Here's the drawing with two shaded views (mm, measured from the low corner). I have some questions. Round coordinates to 2 decimals unless told otherwise and drop trailing zeros. Loops run counter-clockwise (first coordinate to the right, second up) from the corner with the lowest first, then second, coordinate; pieces in that order, holes last. Notation, with made-up numbers: (-5, 45.25) -> (51, 45.25) arc R23 ccw to (51, 76.25) -> close; hole circle Ø3 at (75.5, -29). An arc over 180 degrees is marked (long way). Write each question's results on one line, items separated by ' | '. Start each with the question number.
1) Imagine slicing it at C-C, the plane z = 2.15. List the corners of the cut face in (x, y) for me, plus the area to 3 significant figures.
2) Imagine slicing it at B-B, the plane x = 95. List the corners of the cut face in (y, z) for me, plus the area to 3 significant figures.
3) For P1, Ø3.5, axis at x = 5, y = 5, coming from the +Z side, with a flat end and sliding along its axis, tell me the tip position at first contact or that it passes through.
4) Imagine slicing it at A-A, the plane y = 5. List the corners of the cut face in (x, z) for me, plus the area to 3 significant figures.
5) Imagine slicing it at D-D, the plane x = 75. List the corners of the cut face in (y, z) for me, plus the area to 3 significant figures.
6) If I drill on probe 1 along Y at (x, z) = (95, 1.8); probe 2 along X at (y, z) = (50, 0.8); probe 3 along X at (y, z) = (27.5, 2.25), over which ranges is the centre line in solid material (lowest first)?
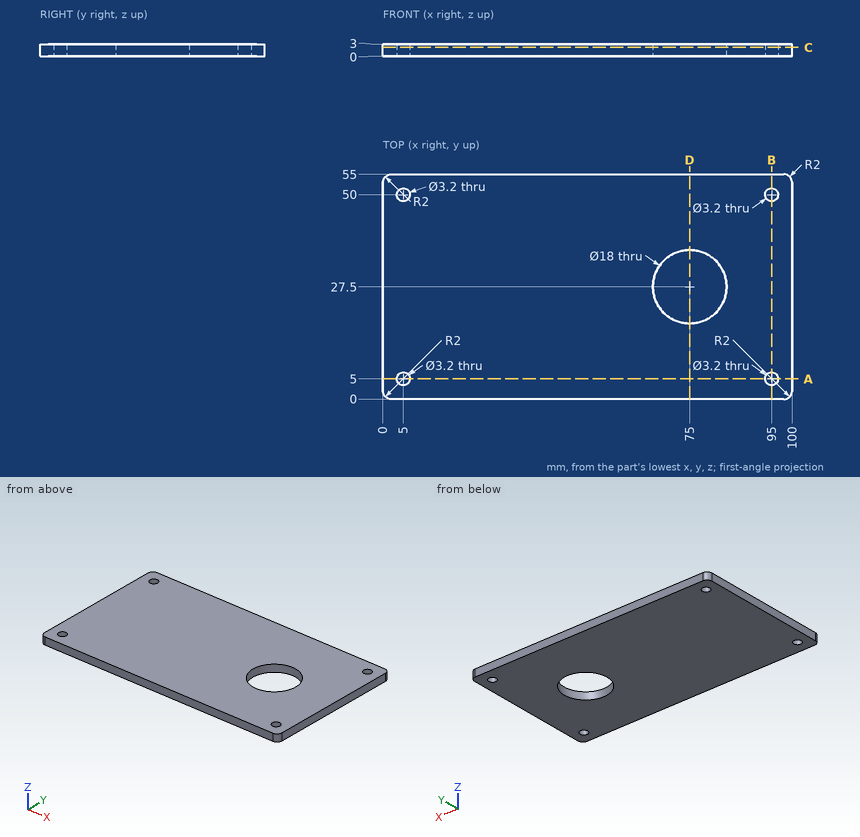
Checked values:
1) outline: (0, 2) arc R2 ccw to (2, 0) -> (98, 0) arc R2 ccw to (100, 2) -> (100, 53) arc R2 ccw to (98, 55) -> (2, 55) arc R2 ccw to (0, 53) -> close; hole circle Ø3.2 at (5, 5); hole circle Ø3.2 at (5, 50); hole circle Ø18 at (75, 27.5); hole circle Ø3.2 at (95, 5); hole circle Ø3.2 at (95, 50) | area: 5,210 mm^2
2) outline: (0, 0) -> (3.4, 0) -> (3.4, 3) -> (0, 3) -> close; (6.6, 0) -> (48.4, 0) -> (48.4, 3) -> (6.6, 3) -> close; (51.6, 0) -> (55, 0) -> (55, 3) -> (51.6, 3) -> close | area: 146 mm^2
3) P1: z = 3
4) outline: (0, 0) -> (3.4, 0) -> (3.4, 3) -> (0, 3) -> close; (6.6, 0) -> (93.4, 0) -> (93.4, 3) -> (6.6, 3) -> close; (96.6, 0) -> (100, 0) -> (100, 3) -> (96.6, 3) -> close | area: 281 mm^2
5) outline: (0, 0) -> (18.5, 0) -> (18.5, 3) -> (0, 3) -> close; (36.5, 0) -> (55, 0) -> (55, 3) -> (36.5, 3) -> close | area: 111 mm^2
6) probe 1: 0 to 3.4, 6.6 to 48.4, 51.6 to 55 | probe 2: 0 to 3.4, 6.6 to 93.4, 96.6 to 100 | probe 3: 0 to 66, 84 to 100
